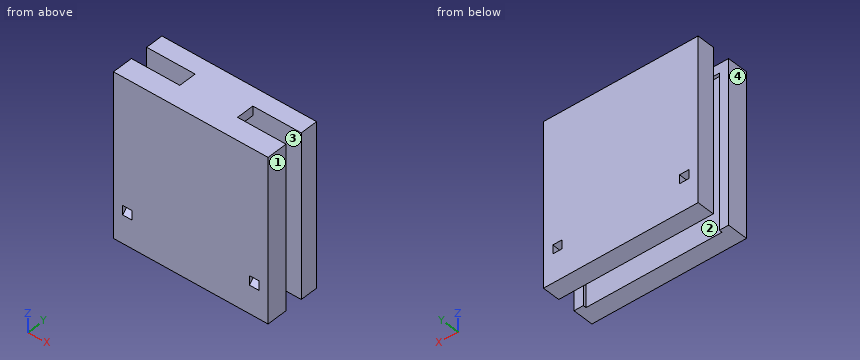
from build123d import *

# Parameters (mm, degrees)
SKETCH1_W           = 9.34
SKETCH1_H           = 3.35
SKETCH1_W_2         = 1.5
SKETCH1_H_2         = 0.5
SKETCH1_W_3         = 6.33
BOSS_EXTRUDE1_DEPTH = 1.5
SKETCH1_6_W         = 1.5
SKETCH1_6_H         = 0.5
BOSS_EXTRUDE4_DEPTH = 25
CAVITY1_START       = -11.015
CAVITY1_DEPTH       = 1.515
CAVITY1_START_2     = 9.485
CAVITY1_2_DEPTH     = 1.515


# Read off the part's stored shape, not the designer's step: Cavity1
with BuildPart() as part:
    # Sketch1 → Boss-Extrude1 (new body)
    with BuildSketch(Plane.XY):
        Rectangle(SKETCH1_W, SKETCH1_H)
        Polygon((11, -1.675), (4.67, -1.675), (-4.67, -1.675), (-11, -1.675), (-12.5, -1.675), (-12.5, -4.525), (12.5, -4.525), (12.5, -1.675), align=None)
        Polygon((-4.67, 1.675), (4.67, 1.675), (12.5, 1.675), (12.5, 4.525), (-12.5, 4.525), (-12.5, 1.675), align=None)
        with Locations((11.75, -1.425)):
            Rectangle(SKETCH1_W_2, SKETCH1_H_2)
        with Locations((7.835, -1.425)):
            Rectangle(SKETCH1_W_3, SKETCH1_H_2)
        with Locations((-11.75, -1.425)):
            Rectangle(SKETCH1_W_2, SKETCH1_H_2)
        with Locations((-7.835, -1.425)):
            Rectangle(SKETCH1_W_3, SKETCH1_H_2)
    extrude(amount=BOSS_EXTRUDE1_DEPTH)

    # Sketch1<6> → Boss-Extrude4 (add)
    with BuildSketch(Plane.XY):
        Polygon((11, -1.675), (4.67, -1.675), (-4.67, -1.675), (-11, -1.675), (-12.5, -1.675), (-12.5, -4.525), (12.5, -4.525), (12.5, -1.675), align=None)
        Polygon((-4.67, 1.675), (4.67, 1.675), (12.5, 1.675), (12.5, 4.525), (-12.5, 4.525), (-12.5, 1.675), align=None)
        with Locations((11.75, -1.425)):
            Rectangle(SKETCH1_6_W, SKETCH1_6_H)
        with Locations((-11.75, -1.425)):
            Rectangle(SKETCH1_6_W, SKETCH1_6_H)
    extrude(amount=-BOSS_EXTRUDE4_DEPTH)

    # Cavity1 outline → Cavity1 (cut)
    with BuildSketch(Plane.YZ.offset(CAVITY1_START)):
        Polygon((-4.525, -18.94), (-4.525, -20.455), (-3.01, -18.94), align=None)
        Polygon((4.525, -18.94), (3.1005, -18.94), (4.525, -20.3645), align=None)
    extrude(amount=CAVITY1_DEPTH, mode=Mode.SUBTRACT)

    # Cavity1 2 outline → Cavity1 2 (cut)
    with BuildSketch(Plane.YZ.offset(CAVITY1_START_2)):
        Polygon((-4.525, -18.94), (-4.525, -20.455), (-3.01, -18.94), align=None)
        Polygon((4.525, -18.94), (3.1005, -18.94), (4.525, -20.3645), align=None)
    extrude(amount=CAVITY1_2_DEPTH, mode=Mode.SUBTRACT)


solid = part.part
The model under review builds one solid part; all positions refer to its coordinate system, in mm. Face numbers are marked on the shaded views. Give positions to 0.01 mm unless a question says otherwise; leave off trailing zeros. Order: outer loops, then holes, each group sorted by start corner. A loop starts at its lowest first (then second) coordinate and runs counter-clockwise, first axis right, second up. Notation, with made-up numbers: M 62,56 L 74,56 A7 ccw 74,64 Z; hole C -27,-17 d8. An arc over 180 degrees is marked long. Use one line per item in the form item = value. Start each with the question number.
Item 1: We need section C-C on x = 4. Give the boundary of the cut face in (y, z) (3 decimals), plus the area to 3 significant figures.
Item 2: We need section B-B on z = -10. Give the boundary of the cut face in (x, y) (3 decimals).
Item 3: To check wall thickness, follow line 1 along Y through (x, z) = (9.5, -11) (3 decimals); line 2 along Z through (x, y) = (3.25, -1.5); line 3 along Y through (x, z) = (11.75, -10.5) (3 decimals). State the ranges of each line that lie inside material, in increasing order. Write a range as from..to.
Item 4: The part is to be moulded in two halves that separate along X. For the marked faces 1, 2, 3 and 4, say which applies: pulls with the +X half, pulls with the -X half, needs draft (parallel to the pull), parting line crosses it, or undercut.
Item 5: We need section D-D on y = 1. Give the boundary of the cut face in (x, z).
Item 6: Insertion check: pin 1 Ø1.7 at (x, y) = (2, 0.5) entering from -Z; pin 2 Ø1.2 at (y, z) = (-0.5, 0.5) entering from -X. Each pin has a flat end and moves straight along its axis. Give the tip position at first contact, or say it passes through.
Item 7: We need section A-A on x = 10.25. Give the boundary of the cut face in (y, z) (1 decimal).
Completed:
q1.outline = M -4.525,-25 L -1.675,-25 L -1.675,0 L 1.675,0 L 1.675,-25 L 4.525,-25 L 4.525,1.5 L -4.525,1.5 Z
q1.area = 156 mm²
q2.outline = M -12.5,-4.525 L 12.5,-4.525 L 12.5,-1.175 L 11,-1.175 L 11,-1.675 L -11,-1.675 L -11,-1.175 L -12.5,-1.175 Z; M -12.5,1.675 L 12.5,1.675 L 12.5,4.525 L -12.5,4.525 Z
q3.line_1 = -4.525..-1.675, 1.675..4.525
q3.line_2 = 0..1.5
q3.line_3 = -4.525..-1.175, 1.675..4.525
q4.face_1 = pulls with the +X half
q4.face_2 = undercut
q4.face_3 = needs draft
q4.face_4 = pulls with the -X half
q5.outline = M -4.67,0 L 4.67,0 L 4.67,1.5 L -4.67,1.5 Z
q6.pin_1 = 0
q6.pin_2 = -4.67
q7.outline = M -4.5,-25 L -1.7,-25 L -1.7,0 L -1.2,0 L -1.2,1.5 L -4.5,1.5 L -4.5,-18.9 L -3,-18.9 L -4.5,-20.5 Z; M 1.7,-25 L 4.5,-25 L 4.5,-20.4 L 3.1,-18.9 L 4.5,-18.9 L 4.5,1.5 L 1.7,1.5 Z
